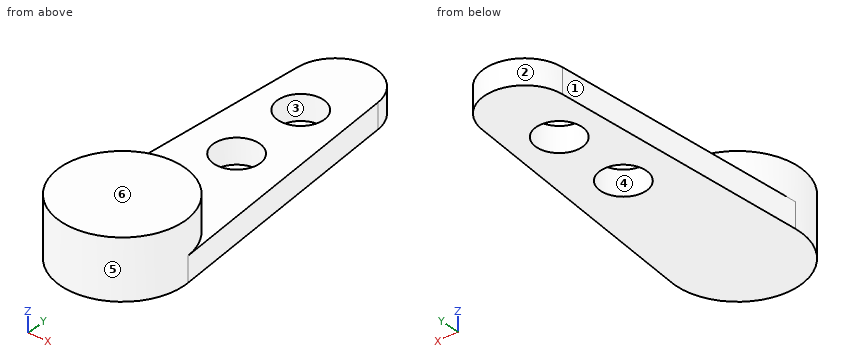
```python
from build123d import *

# Parameters (mm, degrees)
F1_DEPTH = 1.81
F2_DEPTH = 4.3
F4_D     = 3.3


with BuildPart() as f1:
    # F0 (on Top) → F1 (new body)
    with BuildSketch(Plane.XY):
        with BuildLine():
            ThreePointArc((-4.4353227912, 0.3611256545), (0, 4.45), (4.4353227912, 0.3611256545))
            Line((4.4353227912, 0.3611256545), (2.8904350774, 19.3353403141))
            ThreePointArc((2.8904350774, 19.3353403141), (0, 22), (-2.8904350774, 19.3353403141))
            Line((-2.8904350774, 19.3353403141), (-4.4353227912, 0.3611256545))
        make_face()
        with BuildLine():
            ThreePointArc((-4.4353227912, 0.3611256545), (-0.1807118969, -4.4463291838), (4.45, 0))
            ThreePointArc((4.45, 0), (4.4463291838, 0.1807118969), (4.4353227912, 0.3611256545))
            ThreePointArc((4.4353227912, 0.3611256545), (0, 4.45), (-4.4353227912, 0.3611256545))
        make_face()
    extrude(amount=F1_DEPTH)

    # F0 (on Top) → F2 (join)
    with BuildSketch(Plane.XY):
        with BuildLine():
            ThreePointArc((-4.4353227912, 0.3611256545), (-0.1807118969, -4.4463291838), (4.45, 0))
            ThreePointArc((4.45, 0), (4.4463291838, 0.1807118969), (4.4353227912, 0.3611256545))
            ThreePointArc((4.4353227912, 0.3611256545), (0, 4.45), (-4.4353227912, 0.3611256545))
        make_face()
    extrude(amount=F2_DEPTH)

    # F4 (through all)
    with Locations(Plane(origin=(0, 0, 0), x_dir=(1, 0, 0), z_dir=(0, 0, -1))):
        with Locations((0, -10.25), (0, -16)):
            Hole(F4_D / 2)


solid = f1.part
```
Here's how the part is built. I have some questions about the finished solid (model axes, mm). Face numbers are marked on the shaded views. A direction names the side the tool comes from. Round coordinates to 2 decimals unless told otherwise and drop trailing zeros. Loops run counter-clockwise (first coordinate to the right, second up) from the corner with the lowest first, then second, coordinate; pieces in that order, holes last. Notation, with made-up numbers: (-27.5, 16.5) -> (-8.5, 16.5) arc R20 cw to (-8.5, 42.5) -> close; hole circle Ø7 at (4.5, 33). An arc over 180 degrees is marked (long way). Answer as CSV lines item,"result".
1. Thinking about a two-plate mould opening in X: for the marked faces 1, 2, 3 and 4, which applies, released by +X, released by -X, zero draft, split by the parting line, or undercut?
Final values:
face 1,"released by -X"
face 2,"split by the parting line"
face 3,"undercut"
face 4,"undercut"
2. If we section it at D-D on y = 1: Please give me the cut outline in (x, z), plus the area to 3 significant figures.
Final values:
outline,"(-4.38, 0) -> (4.38, 0) -> (4.38, 1.81) -> (4.34, 1.81) -> (4.34, 4.3) -> (-4.34, 4.3) -> (-4.34, 1.81) -> (-4.38, 1.81) -> close"
area,"37.5 mm^2"
3. If we section it at A-A on x = 0.5: Please give me the cut outline in (y, z).
Final values:
outline,"(-4.42, 0) -> (8.68, 0) -> (8.68, 1.81) -> (4.42, 1.81) -> (4.42, 4.3) -> (-4.42, 4.3) -> close; (11.82, 0) -> (14.43, 0) -> (14.43, 1.81) -> (11.82, 1.81) -> close; (17.57, 0) -> (21.96, 0) -> (21.96, 1.81) -> (17.57, 1.81) -> close"
4. If we section it at C-C on z = 1.55: Please give me the cut outline in (x, y).
Final values:
outline,"(-4.44, 0.36) arc R4.45 ccw (long way) to (4.44, 0.36) -> (2.89, 19.34) arc R2.9 ccw to (-2.89, 19.34) -> close; hole circle Ø3.3 at (0, 10.25); hole circle Ø3.3 at (0, 16)"
5. If we section it at B-B on y = 10.25: Please give me the cut outline in (x, z).
Final values:
outline,"(-3.63, 0) -> (-1.65, 0) -> (-1.65, 1.81) -> (-3.63, 1.81) -> close; (1.65, 0) -> (3.63, 0) -> (3.63, 1.81) -> (1.65, 1.81) -> close"
6. If I drill on L1, parallel to Y at x = 0, z = 1.35; L2, parallel to Y at x = -1.25, z = 1.45; L3, parallel to Z at x = -3.25, y = 8, over which ranges is the centre line in solid material (lowest first)?
Final values:
L1,"y = -4.45 to 8.6, 11.9 to 14.35, 17.65 to 22"
L2,"y = -4.27 to 9.17, 11.33 to 14.92, 17.08 to 21.72"
L3,"z = 0 to 1.81"
7. Which directions (+Z, -Z, +X, -X, +Y, -Y) give clear straight access to the entire face, cutting with the end or side of a thin tool? Please do the marked faces 5 and 6.
Final values:
face 5,"+Z"
face 6,"+Z, +X, -X, +Y, -Y"
8. For pin 1 (2 mm diameter, centred on x = -0.5, z = 2, fed in from -Y); pin 2 (1 mm diameter, centred on y = 11, z = 3.5, fed in from -X); pin 3 (2.5 mm diameter, centred on x = -1, y = 9.5, fed in from +Z), each with a flat end and sliding along its axis, tell me the tip position at first contact or that it passes through.
Final values:
pin 1,"stops at y = -4.45"
pin 2,"passes through"
pin 3,"stops at z = 1.81"
